Study the drawing (mm; zero at the part's minimum x, y, z) and answer. A direction names the side the tool comes from. Round coordinates to 2 decimals unless told otherwise and drop trailing zeros. Write each loop counter-clockwise with the first axis right and the second up, starting at its lowest first coordinate (ties: lowest second). Pieces come first, ordered by that corner, then holes. Notation, with made-up numbers: M 13,72 L 25,72 A28 ccw 25,97 Z; hole C 59.25,37 d1. An arc over 180 degrees is marked long. Put each result on its own line as item: value. Start each with the question number.
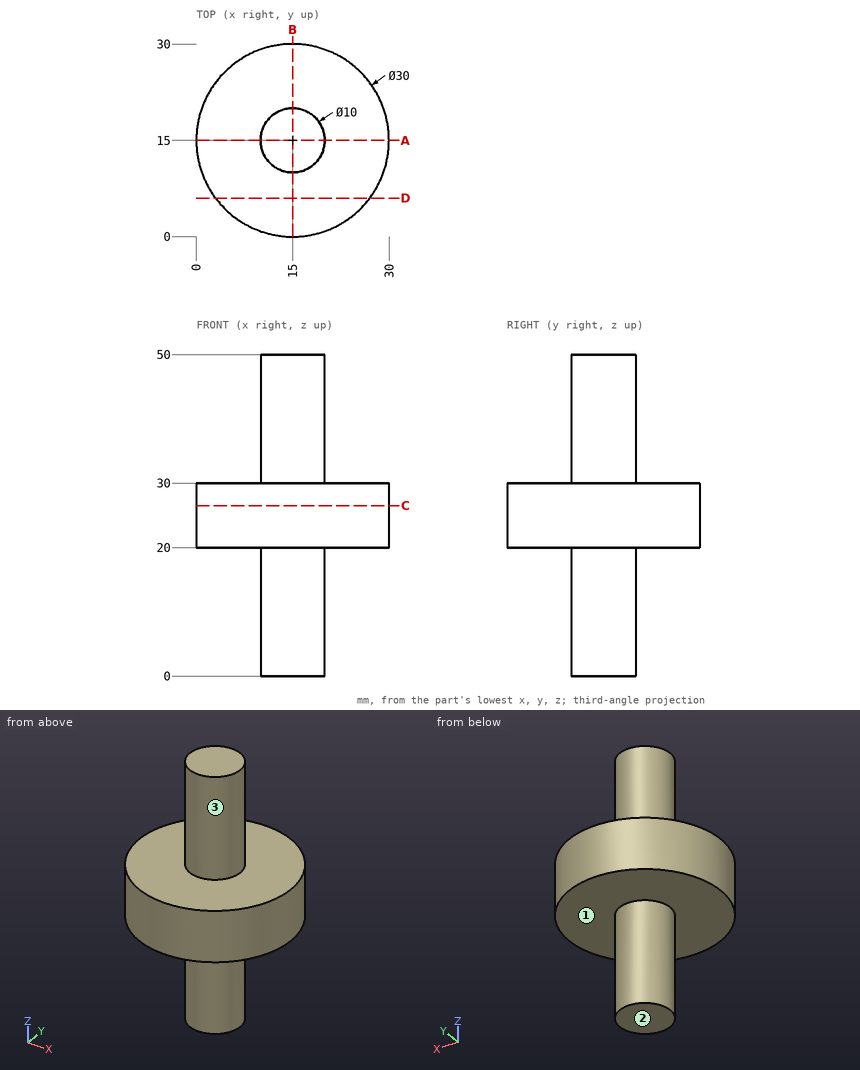
Item 1: Section D-D (y = 6) is taken. Give the vertices of the cut face in (x, z).
Item 2: Consider line 1 along Z through (x, y) = (28.75, 16.25); line 2 along X through (y, z) = (14.75, 25); line 3 along X through (y, z) = (18.75, 17). Determine where each line is inside the solid, lowest interval first. Write a range as [from, to].
Item 3: Flat-ended cylindrical pins translate along their axes: pin 1 (2 mm diameter, centred on x = 8.5, y = 23, fed in from +Z); pin 2 (3 mm diameter, centred on x = 24, y = 12, fed in from -Z); pin 3 (8 mm diameter, centred on y = 17, z = 40, fed in from +X); pin 4 (1.5 mm diameter, centred on x = 24.5, z = 18.5, fed in from -Y). Find the tip coordinate at first contact, or state that the pin passes through.
Item 4: Section A-A (y = 15) is taken. Give the vertices of the cut face in (x, z), and give its area (3 significant figures).
Item 5: Section C-C (z = 26.5) is taken. Give the vertices of the cut face in (x, y), and give its area (3 significant figures).
Item 6: Which of the six approach directions +Z, -Z, +X, -X, +Y, -Y give full straight-line access (tool end or side, diameter ignored) to the marked faces 1, 2 and 3?
Output values:
1. outline: M 3,20 L 27,20 L 27,30 L 3,30 Z
2. line 1: z = [20, 30]
2. line 2: x = [0, 30]
2. line 3: x = [11.69, 18.31]
3. pin 1: stops at z = 30
3. pin 2: stops at z = 20
3. pin 3: stops at x = 20
3. pin 4: passes through
4. outline: M 0,20 L 10,20 L 10,0 L 20,0 L 20,20 L 30,20 L 30,30 L 20,30 L 20,50 L 10,50 L 10,30 L 0,30 Z
4. area: 700 mm^2
5. outline: C 15,15 d30
5. area: 707 mm^2
6. face 1: -Z
6. face 2: -Z, +X, -X, +Y, -Y
6. face 3: +Z
